Build history of the part. All positions in model axes, mm. A direction names the side the tool comes from. Give positions to 0.01 mm unless a question says otherwise; leave off trailing zeros. Order: outer loops, then holes, each group sorted by start corner. A loop starts at its lowest first (then second) coordinate and runs counter-clockwise, first axis right, second up. Notation, with made-up numbers: M 87.5,88 L 136.5,88 A18 cw 136.5,101 Z; hole C -21.75,57 d10. An arc over 180 degrees is marked long. Use CSV: the item, a comma, the result in double quotes. Start each with the question number.
Item 1: Band-saw the part on A-A on y = 17.5. Write the cut outline in (x, z) (3 decimals), plus the area to 3 significant figures.
Item 2: Band-saw the part on B-B on z = 2.75. Give the number of separate pieces and of enclosed holes in the cut face, plus the area to 3 significant figures.
Item 3: Two-plate mould, pull along X, no slides. Class faces 5 (the cylindrical face through (5.59, 16.55, 1.48)), 6 (the cylindrical face through (2.2, 13, 1.2)), 7 (the cylindrical face through (3.68, 27.75, 1.48)), 8 (the cylindrical face through (6.66, 23.75, 1.23)): pulls with the +X half, pulls with the -X half, needs draft (parallel to the pull), parting line crosses it, or undercut.
Item 4: Wall check: line 1 along X through (y, z) = (19.75, 2.4) (3 decimals); line 2 along Y through (x, z) = (2.75, 0.2); line 3 along Y through (x, z) = (3.25, 0.4). Give the ranges that are in metal, low to high.
Item 5: Pin check, flat tips, straight feed: P1, Ø1.5, axis at x = 6.5, z = 1.5, coming from the +Y side; P2, Ø1.5, axis at x = 7.5, y = 11, coming from the -Z side; P3, Ø1.5, axis at y = 20.5, z = 1, coming from the -X side (3 decimals); P4, Ø1.5, axis at y = 8, z = 0.5, coming from the +X side. Stop position of each tip, or through.
Item 6: Which spindle directions (+Z, -Z, +X, -X, +Y, -Y) get a long thin tool onto all of the face, cutting with end or side? Do faces 1 (the flat face through (7.375, 20, 1)), 2 (the cylindrical face through (6.69, 11.84, 1.23)), 3 (the cylindrical face through (0.583, 11.865, 1.232)), 4 (the flat face through (1.375, 20, 1)). Say none if no direction does.
from build123d import *

# Parameters (mm, degrees)
F0_R     = 1
F1_DEPTH = 3
F2_R     = 0.5


with BuildPart() as f1:
    # F0 (on Top) → F1 (new body)
    with BuildSketch(Plane.XY):
        with BuildLine():
            Line((-0.125, 22), (-0.125, 17.25))
            ThreePointArc((-0.125, 17.25), (0.370541, 15.755964), (1.660714, 14.854213))
            ThreePointArc((1.660714, 14.854213), (2.176784, 14.493512), (2.375, 13.895898))
            Line((2.375, 13.895898), (2.375, 13.567332))
            ThreePointArc((2.375, 13.567332), (2.187046, 12.983739), (1.693838, 12.619523))
            ThreePointArc((1.693838, 12.619523), (0.570596, 11.850719), (0.016613, 10.607402))
            Line((0.016613, 10.607402), (-1.319498, 1.357402))
            ThreePointArc((-1.319498, 1.357402), (-0.735085, -0.636535), (1.154823, -1.5))
            Line((1.154823, -1.5), (6.095177, -1.5))
            ThreePointArc((6.095177, -1.5), (7.985085, -0.636535), (8.569498, 1.357402))
            Line((8.569498, 1.357402), (7.233387, 10.607402))
            ThreePointArc((7.233387, 10.607402), (6.679404, 11.850719), (5.556162, 12.619523))
            ThreePointArc((5.556162, 12.619523), (5.062954, 12.983739), (4.875, 13.567332))
            Line((4.875, 13.567332), (4.875, 13.895898))
            ThreePointArc((4.875, 13.895898), (5.073216, 14.493512), (5.589286, 14.854213))
            ThreePointArc((5.589286, 14.854213), (6.879459, 15.755964), (7.375, 17.25))
            Line((7.375, 17.25), (7.375, 22))
            ThreePointArc((7.375, 22), (6.642767, 23.767767), (4.875, 24.5))
            Line((4.875, 24.5), (4.774049, 24.975951))
            ThreePointArc((4.774049, 24.975951), (3.625, 27.75), (2.475951, 24.975951))
            Line((2.475951, 24.975951), (2.375, 24.5))
            ThreePointArc((2.375, 24.5), (0.607233, 23.767767), (-0.125, 22))
        make_face()
        with BuildLine():
            Line((6.095177, 0), (1.154823, 0))
            ThreePointArc((1.154823, 0), (0.398859, 0.345386), (0.165094, 1.142961))
            Line((0.165094, 1.142961), (1.501205, 10.392961))
            ThreePointArc((1.501205, 10.392961), (1.83632, 11.005963), (2.490934, 11.25))
            Line((2.490934, 11.25), (3.625, 11.25))
            Line((3.625, 11.25), (4.759066, 11.25))
            ThreePointArc((4.759066, 11.25), (5.41368, 11.005963), (5.748795, 10.392961))
            Line((5.748795, 10.392961), (7.084906, 1.142961))
            ThreePointArc((7.084906, 1.142961), (6.851141, 0.345386), (6.095177, 0))
        make_face(mode=Mode.SUBTRACT)
        with BuildLine():
            Line((4.875, 16.25), (3.625, 16.25))
            Line((3.625, 16.25), (2.375, 16.25))
            ThreePointArc((2.375, 16.25), (1.667893, 16.542893), (1.375, 17.25))
            Line((1.375, 17.25), (1.375, 22))
            ThreePointArc((1.375, 22), (1.667893, 22.707107), (2.375, 23))
            Line((2.375, 23), (4.875, 23))
            ThreePointArc((4.875, 23), (5.582107, 22.707107), (5.875, 22))
            Line((5.875, 22), (5.875, 17.25))
            ThreePointArc((5.875, 17.25), (5.582107, 16.542893), (4.875, 16.25))
        make_face(mode=Mode.SUBTRACT)
        with Locations((3.625, 26.125)):
            Circle(F0_R, mode=Mode.SUBTRACT)
    extrude(amount=F1_DEPTH)

    # F2
    f2_edges = [f1.edges().sort_by_distance(p)[0] for p in [
        (7.901443, 5.982402, 3),
    ]]
    fillet(f2_edges, radius=F2_R)


solid = f1.part
Model answer:
1,outline,"M -0.125,0 L 1.375,0 L 1.375,3 L 0.375,3 A0.5 ccw -0.125,2.5 Z; M 5.875,0 L 7.375,0 L 7.375,2.5 A0.5 ccw 6.875,3 L 5.875,3 Z"
1,area,"8.89 mm^2"
2,separate pieces,"1"
2,enclosed holes,"3"
2,area,"100 mm^2"
3,face 5,"undercut"
3,face 6,"pulls with the -X half"
3,face 7,"parting line crosses it"
3,face 8,"pulls with the +X half"
4,line 1,"x = -0.125 to 1.375, 5.875 to 7.375"
4,line 2,"y = -1.5 to 0, 11.25 to 16.25, 23 to 25.64, 26.61 to 27.49"
4,line 3,"y = -1.5 to 0, 11.25 to 16.25, 23 to 25.2, 27.05 to 27.71"
5,P1,"stops at y = 24.34"
5,P2,"stops at z = 0"
5,P3,"stops at x = -0.125"
5,P4,"stops at x = 7.72"
6,face 1,"+Z, -Z, +X, +Y"
6,face 2,"+Z, -Z, +X"
6,face 3,"+Z, -Z, -X"
6,face 4,"+Z, -Z"
